CAD build for the part. Positions are in the model's coordinates, mm. Face numbers are marked on the shaded views. Round coordinates to 2 decimals unless told otherwise and drop trailing zeros. Write each loop counter-clockwise with the first axis right and the second up, starting at its lowest first coordinate (ties: lowest second). Pieces come first, ordered by that corner, then holes. Notation, with made-up numbers: (50.25, -22.75) - (54.25, -22.75) arc R24 cw to (54.25, -0.75) - close; hole circle Ø10 at (39.25, 36.5). An arc over 180 degrees is marked (long way). Answer in a Markdown table with one row per item.
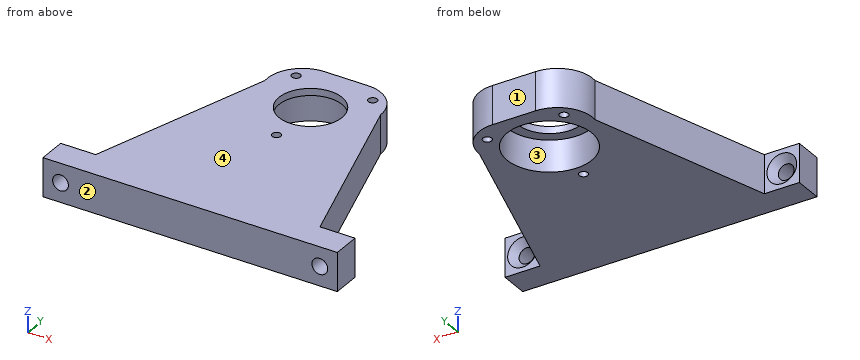
```python
from build123d import *

# Parameters (mm, degrees)
SCHIZZO1_R                   = 12.1
ESTRUSIONE_ESTRUSIONE1_DEPTH = 11
ESTRUSIONE_ESTRUSIONE2_START = -2
SCHIZZO2_R                   = 12.1
SCHIZZO2_R_2                 = 9
ESTRUSIONE_ESTRUSIONE2_DEPTH = 2
SCHIZZO3_R                   = 2.25
TAGLIO_ESTRUSIONE1_DEPTH     = 77.182412669
SMUSSO1_SIZE                 = 2
SCHIZZO4_R                   = 1.25
TAGLIO_ESTRUSIONE2_DEPTH     = 70.679623994


with BuildPart() as part:
    # Schizzo1 → Estrusione-Estrusione1 (new body)
    with BuildSketch(Plane.XY):
        with BuildLine():
            Line((-6.171311325, 16.1), (6.171311325, 16.1))
            ThreePointArc((6.171311325, 16.1), (13.242379137, 13.171067812), (16.171311325, 6.1))
            Line((16.171311325, 6.1), (32, -46.5))
            Line((32, -46.5), (42, -46.5))
            Line((42, -46.5), (42, -54.5))
            Line((42, -54.5), (17, -54.5))
            Line((17, -54.5), (-17, -54.5))
            Line((-17, -54.5), (-42, -54.5))
            Line((-42, -54.5), (-42, -46.5))
            Line((-42, -46.5), (-32, -46.5))
            Line((-32, -46.5), (-16.1, 4.907883736))
            ThreePointArc((-16.1, 4.907883736), (-13.651991863, 12.73622021), (-6.171311325, 16.1))
        make_face()
        Circle(SCHIZZO1_R, mode=Mode.SUBTRACT)
    extrude(amount=ESTRUSIONE_ESTRUSIONE1_DEPTH)

    # Schizzo2 → Estrusione-Estrusione2 (add)
    with BuildSketch(Plane.XY.offset(11).offset(ESTRUSIONE_ESTRUSIONE2_START)):
        Circle(SCHIZZO2_R)
        Circle(SCHIZZO2_R_2, mode=Mode.SUBTRACT)
    extrude(amount=ESTRUSIONE_ESTRUSIONE2_DEPTH)

    # Schizzo3 → Taglio-Estrusione1 (cut, through all)
    with BuildSketch(Plane(origin=(0, -46.5, 0), x_dir=(1, 0, 0), z_dir=(0, 1, 0))):
        with Locations(Location((37, -5.5, 0), (0, 0, 270))):
            Circle(SCHIZZO3_R)
        with Locations(Location((-37, -5.5, 0), (0, 0, 270))):
            Circle(SCHIZZO3_R)
    extrude(amount=-TAGLIO_ESTRUSIONE1_DEPTH, mode=Mode.SUBTRACT)

    # Smusso1
    smusso1_edges = [part.edges().sort_by_distance(p)[0] for p in [
        (37, -46.5, 3.25),
        (-37, -46.5, 3.25),
    ]]
    chamfer(smusso1_edges, length=SMUSSO1_SIZE)

    # Schizzo4 → Taglio-Estrusione2 (cut, through all)
    with BuildSketch(Plane(origin=(0, 0, 0), x_dir=(-1, 0, 0), z_dir=(0, 0, -1))):
        with Locations((-10.910719744, 10.851964601)):
            Circle(SCHIZZO4_R)
        with Locations((10.944459062, 10.817992606)):
            Circle(SCHIZZO4_R)
        with Locations((0, -15.38859776)):
            Circle(SCHIZZO4_R)
    extrude(amount=-TAGLIO_ESTRUSIONE2_DEPTH, mode=Mode.SUBTRACT)


solid = part.part
```
Q1. Flat gauge pins, fed straight in: pin 1 (6 mm diameter, centred on y = -20, z = 9.5, fed in from +X); pin 2 (12 mm diameter, centred on x = 3, y = 1, fed in from -Z); pin 3 (5 mm diameter, centred on x = 35.5, z = 4.5, fed in from +Y). Where does each tip first touch, or does it go through?
Computed:
| item | result |
|---|---|
| pin 1 | stops at x = 24.93 |
| pin 2 | stops at z = 9 |
| pin 3 | stops at y = -46.5 |
Q2. Drill centre lines: line 1 (Y direction, x = 0, z = 6.75); line 2 (X direction, y = -52.15, z = 5.5); line 3 (Y direction, x = 0, z = 10.4). Where is each one in solid material? Low to high.
Computed:
| item | result |
|---|---|
| line 1 | y = -54.5 to -16.64, -14.14 to -12.1, 12.1 to 16.1 |
| line 2 | x = -42 to -39.25, -34.75 to 34.75, 39.25 to 42 |
| line 3 | y = -54.5 to -16.64, -14.14 to -9, 9 to 16.1 |
Q3. Pull direction Y, two halves, no side cores. Call the marked faces 1, 2, 3 and 4: released by +Y, released by -Y, zero draft, split by the parting line, or undercut.
Computed:
| item | result |
|---|---|
| face 1 | released by +Y |
| face 2 | released by -Y |
| face 3 | undercut |
| face 4 | zero draft |
Q4. Saw through at B-B on x = 37. List the corners of the cut face in (y, z).
Computed:
| item | result |
|---|---|
| outline | (-54.5, 0) - (-46.5, 0) - (-46.5, 1.25) - (-48.5, 3.25) - (-54.5, 3.25) - close; (-54.5, 7.75) - (-48.5, 7.75) - (-46.5, 9.75) - (-46.5, 11) - (-54.5, 11) - close |
Q5. Saw through at C-C on x = 0. List the corners of the cut face in (y, z), then the cut area to 3 significant figures.
Computed:
| item | result |
|---|---|
| outline | (-54.5, 0) - (-16.64, 0) - (-16.64, 11) - (-54.5, 11) - close; (-14.14, 0) - (-12.1, 0) - (-12.1, 9) - (-9, 9) - (-9, 11) - (-14.14, 11) - close; (9, 9) - (12.1, 9) - (12.1, 0) - (16.1, 0) - (16.1, 11) - (9, 11) - close |
| area | 495 mm2 |
Q6. Saw through at A-A on z = 5.5. List the corners of the cut face in (x, y).
Computed:
| item | result |
|---|---|
| outline | (-42, -54.5) - (-39.25, -54.5) - (-39.25, -48.5) - (-41.25, -46.5) - (-42, -46.5) - close; (-34.75, -54.5) - (34.75, -54.5) - (34.75, -48.5) - (32.75, -46.5) - (32, -46.5) - (16.17, 6.1) arc R10 ccw to (6.17, 16.1) - (-6.17, 16.1) arc R10 ccw to (-16.1, 4.91) - (-32, -46.5) - (-32.75, -46.5) - (-34.75, -48.5) - close; (39.25, -54.5) - (42, -54.5) - (42, -46.5) - (41.25, -46.5) - (39.25, -48.5) - close; hole circle Ø2.5 at (-10.94, 10.82); hole circle Ø24.2 at (0, 0); hole circle Ø2.5 at (0, -15.39); hole circle Ø2.5 at (10.91, 10.85) |
Q7. Saw through at D-D on y = -44. List the corners of the cut face in (x, z).
Computed:
| item | result |
|---|---|
| outline | (-31.23, 0) - (31.25, 0) - (31.25, 11) - (-31.23, 11) - close |
